from build123d import *

# Parameters (mm, degrees)
SKETCH4_R           = 13.7795
BOSS_EXTRUDE1_DEPTH = 25.4
SKETCH5_R           = 13.7795
BOSS_EXTRUDE2_DEPTH = 12.7


with BuildPart() as part:
    # Sketch1 → Revolve1 (revolve)
    with BuildSketch(Plane.XY):
        Polygon((-31.75, -13.7795), (-12.7, -13.7795), (-12.7, -10.6172), (-31.75, -10.7696), align=None)
        Polygon((31.75, -10.7696), (12.7, -10.6172), (12.7, -13.7795), (31.75, -13.7795), align=None)
    revolve(axis=Axis((-31.75, 0, 0), (1, 0, 0)))



with BuildPart() as body_2:
    # Sketch2 → Revolve2 (revolve)
    with BuildSketch(Plane.XY):
        Polygon((10.7696, 31.75), (10.6172, 12.7), (13.7795, 12.7), (13.7795, 31.75), align=None)
    revolve(axis=Axis((0, 0, 0), (0, 1, 0)))


with BuildPart() as part_1:
    add(part.part)

    add(body_2.part)  # Boss-Extrude1 merges body 2
    # Sketch4 → Boss-Extrude1 (add)
    with BuildSketch(Plane(origin=(-12.7, 0, 0), x_dir=(0, 0, -1), z_dir=(1, 0, 0))):
        Circle(SKETCH4_R)
    extrude(amount=BOSS_EXTRUDE1_DEPTH)

    # Sketch5 → Boss-Extrude2 (add)
    with BuildSketch(Plane.XZ.offset(-12.7)):
        Circle(SKETCH5_R)
    extrude(amount=BOSS_EXTRUDE2_DEPTH)

    # Sketch6 → Cut-Revolve1 (revolve, cut)
    with BuildSketch(Plane.XY):
        Polygon((-31.75, -10.7696), (-12.7, -10.6172), (-12.7, -7.8994), (12.7, -7.8994), (12.7, -10.6172), (31.75, -10.7696), (31.75, 0), (-31.75, 0), align=None)
    revolve(axis=Axis((31.75, 0, 0), (-1, 0, 0)), mode=Mode.SUBTRACT)

    # Sketch7 → Cut-Revolve2 (revolve, cut)
    with BuildSketch(Plane.XY):
        Polygon((10.7696, 31.75), (10.6172, 12.7), (7.8994, 12.7), (7.8994, 0), (0, 0), (0, 31.75), align=None)
    revolve(axis=Axis((0, 0, 0), (0, 1, 0)), mode=Mode.SUBTRACT)


solid = part_1.part
Geometry: final body of the model. Coordinates: model frame, mm. Give positions to 0.01 mm unless a question says otherwise; leave off trailing zeros. Write each loop counter-clockwise with the first axis right and the second up, starting at its lowest first coordinate (ties: lowest second). Pieces come first, ordered by that corner, then holes.
(1) First-contact query: P1, Ø9.5, axis at y = 0, z = 0, coming from the +X side; P2, Ø4, axis at x = 4, z = -7.5, coming from the +Y side; P3, Ø1, axis at x = 1, z = -3.5, coming from the -Y side; P4, Ø5.5, axis at y = 7, z = 2, coming from the -X side. Flat tips, straight axial feed; report the tip coordinate or a pass-through.
(2) Cut plane A-A, the plane z = 4.25. Give the number of separate pieces and of enclosed holes in the cut face, then the cut area to 3 significant figures.
(3) Ray query, line 1 (X direction, y = 8.5, z = 0); line 2 (Z direction, x = -5, y = 0); line 3 (X direction, y = 24.5, z = 12.5). Return the intervals inside material, ascending.
(4) Mould query, pull axis X, two halves, no side actions, for faces 1 (the flat face through (31.75, -6.1, 9.1)), 2 (the cylindrical face through (7.535, 9.083, -2.373)), 3 (the cylindrical face through (-10.16, 19.63, 9.31)). Classes: released by +X, released by -X, zero draft, split by the parting line, or undercut.
(5) Cut plane B-B, the plane x = -18. Return loops of the section in (y, z).
(6) Cut plane C-C, the plane y = 15. Return loops of the section in (x, z).
Values follow:
1. P1: passes through
1. P2: stops at y = 12.7
1. P3: stops at y = -13.45
1. P4: stops at x = -12.7
2. separate pieces: 3
2. enclosed holes: 0
2. area: 613 mm2
3. line 1: x = -12.7 to -7.9, 7.9 to 12.7
3. line 2: z = -13.78 to -7.9, 7.9 to 13.78
3. line 3: x = -5.8 to 5.8
4. face 1: released by +X
4. face 2: undercut
4. face 3: split by the parting line
5. outline: circle Ø27.56 at (0, 0); hole circle Ø21.32 at (0, 0)
6. outline: circle Ø27.56 at (0, 0); hole circle Ø21.27 at (0, 0)
